```python
from build123d import *

# Parameters (mm, degrees)
MAIN_W                  = 20
MAIN_H                  = 34
MAIN_R                  = 1.5
MAIN_EXTRUSION_DEPTH    = 20
ESQUISSE2_R             = 2.25
ENL_V_MAT_EXTRU_1_DEPTH = 45.226688775
ESQUISSE3_W             = 10
ESQUISSE3_H             = 10
BOSS_EXTRU_3_DEPTH      = 50
ESQUISSE4_W             = 20
ESQUISSE4_H             = 20
BOSS_EXTRU_4_DEPTH      = 3


with BuildPart() as part:
    # Main → Main Extrusion (new body)
    with BuildSketch(Plane.XY):
        with Locations((10, 0)):
            Rectangle(MAIN_W, MAIN_H)
        with Locations((5, 12.5)):
            Circle(MAIN_R, mode=Mode.SUBTRACT)
        with Locations((15, 12.5)):
            Circle(MAIN_R, mode=Mode.SUBTRACT)
        with Locations((5, -12.5)):
            Circle(MAIN_R, mode=Mode.SUBTRACT)
        with Locations((15, -12.5)):
            Circle(MAIN_R, mode=Mode.SUBTRACT)
    extrude(amount=MAIN_EXTRUSION_DEPTH)

    # Esquisse2 → Enlèv. mat.-Extru.1 (cut, through all)
    with BuildSketch(Plane.XZ.offset(17)):
        with Locations(Location((10, 10, 0), (0, 0, 270))):
            Circle(ESQUISSE2_R)
    extrude(amount=-ENL_V_MAT_EXTRU_1_DEPTH, mode=Mode.SUBTRACT)

    # Esquisse3 → Boss.-Extru.3 (add)
    with BuildSketch(Plane.ZY):
        with Locations((5, 0)):
            Rectangle(ESQUISSE3_W, ESQUISSE3_H)
    extrude(amount=BOSS_EXTRU_3_DEPTH)

    # Esquisse4 → Boss.-Extru.4 (add)
    with BuildSketch(Plane.ZY.offset(50)):
        with Locations((10, 0)):
            Rectangle(ESQUISSE4_W, ESQUISSE4_H)
    extrude(amount=BOSS_EXTRU_4_DEPTH)


solid = part.part
```
The listing builds one solid part. Answer for the finished solid, in the listing's coordinates (mm). A direction names the side the tool comes from. Coordinates: 2 decimals unless noted, no trailing zeros. Loops run counter-clockwise (first coordinate to the right, second up) from the corner with the lowest first, then second, coordinate; pieces in that order, holes last. Notation, with made-up numbers: M -4.5,11.5 L 42.5,11.5 A27 ccw 42.5,31.5 Z; hole C -25,36 d3. An arc over 180 degrees is marked long. Answer as a JSON object with one key per item and string values. Group by question number.
Item 1: Determine the mould class of faces 1 (the face through (-53, 0, 10)), 2 (the face through (-25, 5, 5)), 3 (the face through (13.5, 12.57, 9.86)) for opening direction Y: +Y half, -Y half, draft (parallel to the pull), parting line (faces both ways), or undercut.
Item 2: Section A-A (y = -12.5) is taken. Write down the section's boundary in (x, z), and give its area (3 significant figures).
Item 3: Each of these flat-tipped pins is pushed along its axis until it touches: P1, Ø0.9, axis at x = -51.5, z = 10.5, coming from the +Y side; P2, Ø2.5, axis at x = 15, y = 12.5, coming from the -Z side; P3, Ø5, axis at x = -31, y = 2.5, coming from the +Z side; P4, Ø5, axis at x = 10, z = 10, coming from the -Y side. Where does it stop, or does it pass through?
Item 4: Section B-B (z = 8.5) is taken. Write down the section's boundary in (x, y).
Item 5: Section D-D (x = 5) is taken. Write down the section's boundary in (y, z), and give its area (3 significant figures).
Item 6: Consider L1, parallel to Y at x = 15, z = 8.25; L2, parallel to X at y = 13, z = 3.5; L3, parallel to X at y = 6.5, z = 10.25. Determine where each line is inside the solid, lowest interval first.
Item 7: Which of the six approach directions +Z, -Z, +X, -X, +Y, -Y give full straight-line access (tool end or side, diameter ignored) to faces 4 (the face through (0, 0, 12)), 5 (the face through (-51, -10, 10)), 6 (the face through (-51, 10, 10))?
Item 8: Section C-C (z = 2.75) is taken. Write down the section's boundary in (x, y).
Solved:
{
 "1": {"face 1": "draft", "face 2": "+Y half", "face 3": "undercut"},
 "2": {"outline": "M 0,0 L 3.5,0 L 3.5,20 L 0,20 Z; M 6.5,0 L 13.5,0 L 13.5,20 L 6.5,20 Z; M 16.5,0 L 20,0 L 20,20 L 16.5,20 Z; hole C 10,10 d4.5", "area": "264 mm2"},
 "3": {"P1": "stops at y = 10", "P2": "passes through", "P3": "stops at z = 10", "P4": "stops at y = -17"},
 "4": {"outline": "M -53,-10 L -50,-10 L -50,-5 L 0,-5 L 0,-17 L 8.32,-17 L 8.32,17 L 0,17 L 0,5 L -50,5 L -50,10 L -53,10 Z; M 11.68,-17 L 20,-17 L 20,17 L 11.68,17 Z; hole C 5,-12.5 d3; hole C 5,12.5 d3; hole C 15,-12.5 d3; hole C 15,12.5 d3"},
 "5": {"outline": "M -17,0 L -14,0 L -14,20 L -17,20 Z; M -11,0 L 11,0 L 11,20 L -11,20 Z; M 14,0 L 17,0 L 17,20 L 14,20 Z", "area": "560 mm2"},
 "6": {"L1": "y = -17 to -14, -11 to 11, 14 to 17", "L2": "x = 0 to 3.59, 6.41 to 13.59, 16.41 to 20", "L3": "x = -53 to -50, 0 to 7.76, 12.24 to 20"},
 "7": {"face 4": "+Z", "face 5": "+Z, -Z, -X, -Y", "face 6": "+Z, -Z, -X, +Y"},
 "8": {"outline": "M -53,-10 L -50,-10 L -50,-5 L 0,-5 L 0,-17 L 20,-17 L 20,17 L 0,17 L 0,5 L -50,5 L -50,10 L -53,10 Z; hole C 5,-12.5 d3; hole C 5,12.5 d3; hole C 15,-12.5 d3; hole C 15,12.5 d3"}
}
